For this review, use the dimensioned drawing (mm, ordinates from the lowest corner) and the shaded views. Round coordinates to 2 decimals unless told otherwise and drop trailing zeros. Write each loop counter-clockwise with the first axis right and the second up, starting at its lowest first coordinate (ties: lowest second). Pieces come first, ordered by that corner, then holes. Notation, with made-up numbers: (78.25, 45) - (84.25, 45) arc R21 cw to (84.25, 66) - close; hole circle Ø4 at (-34, 65). An arc over 180 degrees is marked (long way). Return JSON: item names as keys, results as strings.
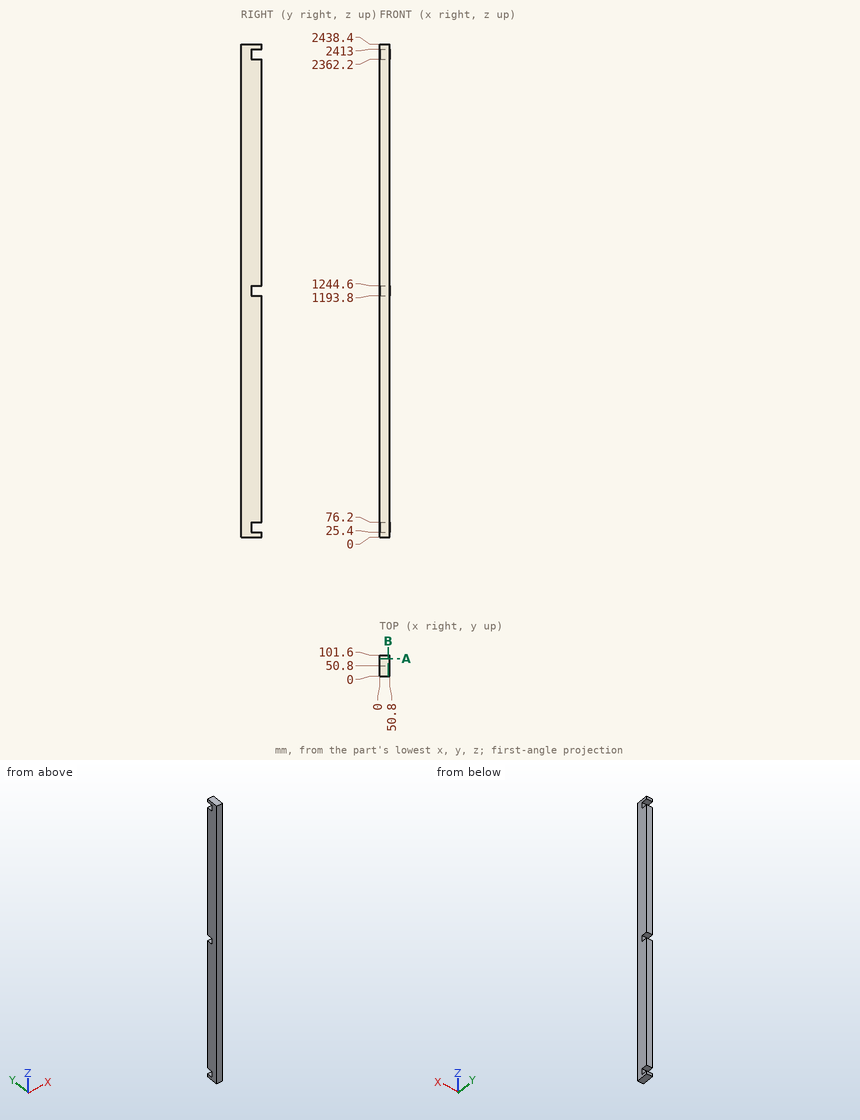
(1) Add section B-B (x = 42). Write out the cut boundary in (y, z), plus the area to 3 significant figures.
Filled in:
{"outline": "(0, 0) - (101.6, 0) - (101.6, 25.4) - (50.8, 25.4) - (50.8, 76.2) - (101.6, 76.2) - (101.6, 1193.8) - (50.8, 1193.8) - (50.8, 1244.6) - (101.6, 1244.6) - (101.6, 2362.2) - (50.8, 2362.2) - (50.8, 2413) - (101.6, 2413) - (101.6, 2438.4) - (0, 2438.4) - close", "area": "240,000 mm2"}
(2) Wall thickness on line 1 (Z direction, x = 42, y = 80); line 2 (Y direction, x = 25, z = 1241.5): over which ranges is each line inside the solid? List them lowest first.
Filled in:
{"line 1": "z = 0 to 25.4, 76.2 to 1193.8, 1244.6 to 2362.2, 2413 to 2438.4", "line 2": "y = 0 to 50.8"}
(3) Add section A-A (y = 85.5). Write out the cut boundary in (x, z).
Filled in:
{"outline": "(0, 0) - (50.8, 0) - (50.8, 25.4) - (0, 25.4) - close; (0, 76.2) - (50.8, 76.2) - (50.8, 1193.8) - (0, 1193.8) - close; (0, 1244.6) - (50.8, 1244.6) - (50.8, 2362.2) - (0, 2362.2) - close; (0, 2413) - (50.8, 2413) - (50.8, 2438.4) - (0, 2438.4) - close"}
(4) Clearance check with a flat-ended pin moving along its axis: pin 1 Ø10 at (x, z) = (25, 684.5) entering from -Y. State where the tip first meets the part, or that it passes through.
Filled in:
{"pin 1": "stops at y = 0"}
